```python
from build123d import *

# Parameters (mm, degrees)
ESQUISSE1_W                    = 25.7
ESQUISSE1_H                    = 34
BOSS_EXTRU_1_DEPTH             = 5.8
ESQUISSE2_W                    = 0.65
ESQUISSE2_H                    = 0.65
BOSS_EXTRU_2_DEPTH             = 6
R_P_TITION_LIN_AIRE1_COUNT     = 5
R_P_TITION_LIN_AIRE1_PITCH     = 2.54
R_P_TITION_LIN_AIRE1_COL_COUNT = 5
R_P_TITION_LIN_AIRE1_COL_PITCH = 2.54


with BuildPart() as part:
    # Esquisse1 → Boss.-Extru.1 (new, symmetric)
    with BuildSketch(Plane.XY):
        Rectangle(ESQUISSE1_W, ESQUISSE1_H)
    extrude(amount=BOSS_EXTRU_1_DEPTH, both=True)

    # Esquisse2 → Boss.-Extru.2 (add)
    with BuildSketch(Plane.XZ.offset(17)):
        with Locations((0, -1.2)):
            Rectangle(ESQUISSE2_W, ESQUISSE2_H)
    boss_extru_2 = extrude(amount=BOSS_EXTRU_2_DEPTH)

    # Répétition linéaire1: Boss.-Extru.2 ×5
    with Locations(*[(i * R_P_TITION_LIN_AIRE1_PITCH, 0, 0) for i in range(1, R_P_TITION_LIN_AIRE1_COUNT)]):
        add(boss_extru_2)

    # Répétition linéaire1 col: Boss.-Extru.2 ×5
    with Locations(*[(-i * R_P_TITION_LIN_AIRE1_COL_PITCH, 0, 0) for i in range(1, R_P_TITION_LIN_AIRE1_COL_COUNT)]):
        add(boss_extru_2)


solid = part.part
```
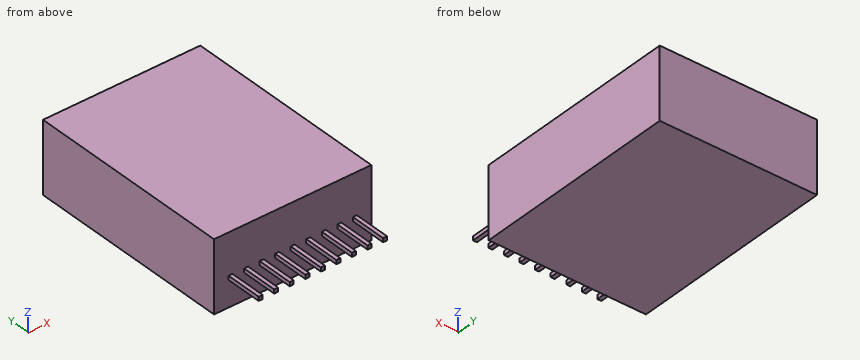
Geometry: final body of the model. Coordinates: model frame, mm. Give positions to 0.01 mm unless a question says otherwise; leave off trailing zeros. Loops run counter-clockwise (first coordinate to the right, second up) from the corner with the lowest first, then second, coordinate; pieces in that order, holes last. Notation, with made-up numbers: (48.25, 53.5) -> (86.25, 53.5) arc R20 cw to (86.25, 76.5) -> close; hole circle Ø8 at (40.5, -30). An arc over 180 degrees is marked (long way). Use one line per item in the form item = value.
Item 1: Section query C-C on x = 1. Output: boundary loops of the cut face in (y, z).
A:
outline = (-17, -5.8) -> (17, -5.8) -> (17, 5.8) -> (-17, 5.8) -> close
Item 2: Section query B-B on z = 4.5. Output: boundary loops of the cut face in (x, y).
A:
outline = (-12.85, -17) -> (12.85, -17) -> (12.85, 17) -> (-12.85, 17) -> close
Item 3: Pin query (flat end, axial travel): P1, Ø0.7, axis at x = -2.5, y = -20.5, coming from the -Z side (3 decimals); P2, Ø3, axis at x = -7.5, z = 3.5, coming from the -Y side; P3, Ø0.7, axis at x = -2.5, y = -20.5, coming from the +Z side (3 decimals). Return the tip coordinate at first contact, or that it passes through.
A:
P1 = -1.525
P2 = -17
P3 = -0.875
Item 4: Line query: probe 1 along Y at (x, z) = (-0.5, -1); probe 2 along Z at (x, y) = (-2.5, -18) (3 decimals). Output: solid intervals per line, ascending.
A:
probe_1 = -17 to 17
probe_2 = -1.525 to -0.875
Item 5: Section query A-A on y = -19. Give the number of separate pieces and of enclosed holes in the cut face, and give its area (3 significant figures).
A:
separate_pieces = 9
enclosed_holes = 0
area = 3.80 mm^2
